Part model, mm, in its own coordinate system. A direction names the side the tool comes from. Coordinates: 2 decimals unless noted, no trailing zeros. Write each loop counter-clockwise with the first axis right and the second up, starting at its lowest first coordinate (ties: lowest second). Pieces come first, ordered by that corner, then holes. Notation, with made-up numbers: (-9, 71.25) - (0, 71.25) arc R10 cw to (0, 90.25) - close; hole circle Ø6 at (31.5, 64.25). An arc over 180 degrees is marked (long way). Write each question's results on one line, items separated by ' | '.
from build123d import *

# Parameters (mm, degrees)
F0_R     = 4.7018325436
F0_W     = 2.4090255611
F0_H     = 3.1813085079
F0_W_2   = 2.413
F0_H_2   = 2.54
F1_DEPTH = 3.175
F2_DEPTH = 9.398
F3_DEPTH = 3.175


# Not quite as in the source:
# - a feature names something its author has since deleted; it is built from what else it names


with BuildPart() as f1:
    # F0 (on Front) → F1 (new body, symmetric)
    with BuildSketch(Plane.XZ):
        with BuildLine():
            ThreePointArc((-13.3044686056, 15.3006398952), (-13.3088027932, 15.5879506834), (-13.3218014117, 15.875))
            ThreePointArc((-13.3218014117, 15.875), (-32.3313565604, 15.9637766028), (-13.49375, 13.4112))
            ThreePointArc((-13.49375, 13.4112), (-13.3519070859, 14.3511912968), (-13.3044686056, 15.3006398952))
        make_face()
        with Locations((-22.8294686056, 15.3006398952)):
            Circle(F0_R, mode=Mode.SUBTRACT)
        with BuildLine():
            Line((-3.96875, 13.4112), (-3.96875, 15.875))
            Line((-3.96875, 15.875), (-13.3218014117, 15.875))
            ThreePointArc((-13.3218014117, 15.875), (-13.3088027932, 15.5879506834), (-13.3044686056, 15.3006398952))
            ThreePointArc((-13.3044686056, 15.3006398952), (-13.3519070859, 14.3511912968), (-13.49375, 13.4112))
            Line((-13.49375, 13.4112), (-3.96875, 13.4112))
        make_face()
        with BuildLine():
            Line((3.96875, -30.1625), (3.96875, 30.1625))
            ThreePointArc((3.96875, 30.1625), (0, 34.13125), (-3.96875, 30.1625))
            Line((-3.96875, 30.1625), (-3.96875, 15.875))
            Line((-3.96875, 15.875), (-3.96875, 13.4112))
            Line((-3.96875, 13.4112), (-3.96875, -30.1625))
            ThreePointArc((-3.96875, -30.1625), (0, -34.13125), (3.96875, -30.1625))
        make_face()
        with Locations((0, -24.1956412792)):
            Rectangle(F0_W, F0_H, mode=Mode.SUBTRACT)
        with Locations((0, 14.4846439362)):
            Rectangle(F0_W_2, F0_H_2, mode=Mode.SUBTRACT)
    extrude(amount=F1_DEPTH, both=True)

    # F0 (on Front) → F2 (join)
    with BuildSketch(Plane.XZ):
        with Locations((0, 14.4846439362)):
            Rectangle(F0_W_2, F0_H_2)
    extrude(amount=F2_DEPTH)

    # F0 (on Front) → F3 (join)
    with BuildSketch(Plane.XZ):
        with Locations((0, 14.4846439362)):
            Rectangle(F0_W_2, F0_H_2)
    extrude(amount=-F3_DEPTH)


solid = f1.part
(1) Saw through at A-A on x = 0. Write the cut outline in (y, z) (3 decimals).
Return value:
outline: (-9.398, 13.215) - (-3.175, 13.215) - (-3.175, -22.605) - (3.175, -22.605) - (3.175, 34.131) - (-3.175, 34.131) - (-3.175, 15.755) - (-9.398, 15.755) - close; (-3.175, -34.131) - (3.175, -34.131) - (3.175, -25.786) - (-3.175, -25.786) - close
(2) Two-plate mould, pull along X, no slides. Class faces 6 (the cylindrical face through (-26.56, 0.04, 12.44)), 7 (the flat face through (0, -9.398, 15)), 8 (the flat face through (-9, 0, 15.875)), 9 (the flat face through (1.206, -6, 14)): released by +X, released by -X, zero draft, split by the parting line, or undercut.
Return value:
face 6: undercut | face 7: zero draft | face 8: undercut | face 9: released by +X
(3) 3-axis set-ups, long thin cutter, end or side, ignore diameter. For faces 1 (the flat face through (0, -6, 15.755)), 2 (the flat face through (-1.206, -6, 14)), 3 (the flat face through (0, -6, 13.215)), 4 (the flat face through (-3.969, 0, -8)), 5 (the flat face through (0, 0, -22.605)): which of +Z, -Z, +X, -X, +Y, -Y reach the whole face in a straight line?
Return value:
face 1: +Z, +X, -X, -Y | face 2: +Z, -Z, -X, -Y | face 3: -Z, +X, -X, -Y | face 4: -Z, +Y, -Y | face 5: +Y, -Y
(4) Saw through at B-B on y = -0.5. Count the separate pieces of the cut face and the enclosed holes in it, then the cut area to 3 significant figures.
Return value:
separate pieces: 1 | enclosed holes: 2 | area: 759 mm^2
(5) Wall check: line 1 (X direction, y = -1.5, z = -24); line 2 (Y direction, x = -19, z = 10.5) (3 decimals); line 3 (X direction, y = 0.5, z = 19.5). Give the ranges that are in metal, low to high. Write a range as from..to.
Return value:
line 1: x = -3.97..-1.2, 1.2..3.97 | line 2: y = -3.175..3.175 | line 3: x = -31.38..-24.94, -20.71..-14.28, -3.97..3.97
(6) Saw through at C-C on x = -21.5. Write the cut outline in (y, z) (3 decimals).
Return value:
outline: (-3.175, 5.869) - (3.175, 5.869) - (3.175, 10.791) - (-3.175, 10.791) - close; (-3.175, 19.811) - (3.175, 19.811) - (3.175, 24.732) - (-3.175, 24.732) - close
(7) Flat gauge pins, fed straight in: P1, Ø1.9, axis at x = -9, y = -1, coming from the +Z side (3 decimals); P2, Ø7, axis at y = -1.5, z = -8.5, coming from the -X side; P3, Ø1.2, axis at x = 0.5, y = -7.5, coming from the +Z side; P4, Ø1.2, axis at x = -0.5, y = 0, coming from the +Z side. Where does each tip first touch, or does it go through?
Return value:
P1: stops at z = 15.875 | P2: stops at x = -3.97 | P3: stops at z = 15.75 | P4: stops at z = 34.13
(8) Saw through at D-D on z = -29. Write the cut outline in (x, y) (3 decimals).
Return value:
outline: (-3.969, -3.175) - (3.969, -3.175) - (3.969, 3.175) - (-3.969, 3.175) - close
